Read the model definition and answer for the solid it produces. Units are mm, in the model's axes. Face numbers are marked on the shaded views. Give positions to 0.01 mm unless a question says otherwise; leave off trailing zeros. Loops run counter-clockwise (first coordinate to the right, second up) from the corner with the lowest first, then second, coordinate; pieces in that order, holes last. Notation, with made-up numbers: (14, -19.5) - (47, -19.5) arc R10 cw to (47, -4.5) - close; hole circle Ø9 at (-40, 52). An arc over 180 degrees is marked (long way). Write item = value, one per line.
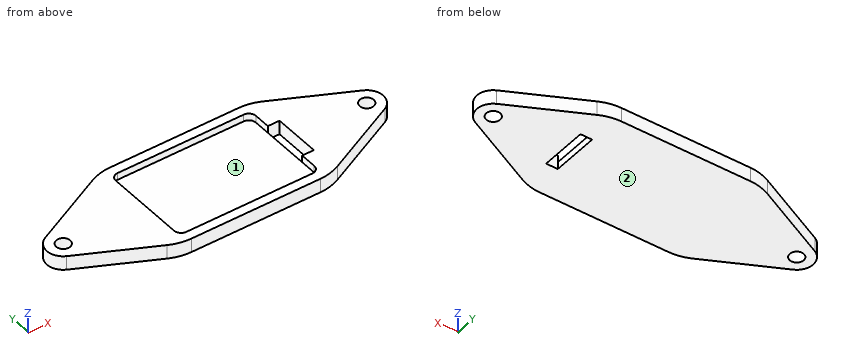
```python
from build123d import *

# Parameters (mm, degrees)
SKETCH1_R           = 1.5
BOSS_EXTRUDE1_DEPTH = 3
BOSS_EXTRUDE2_DEPTH = 1.5


with BuildPart() as part:
    # Sketch1 → Boss-Extrude1 (new body)
    with BuildSketch(Plane.XY):
        with BuildLine():
            Line((-18.151142685, 10.970518354), (-34.046738684, 3.139681424))
            ThreePointArc((-34.046738684, 3.139681424), (-35.999996343, 0.005059225), (-34.055808986, -3.135196708))
            Line((-34.055808986, -3.135196708), (-18.292240263, -10.957704881))
            ThreePointArc((-18.292240263, -10.957704881), (-16.129937386, -11.735939832), (-13.847071731, -12))
            Line((-13.847071731, -12), (13.731889302, -12))
            ThreePointArc((13.731889302, -12), (16.000679339, -11.739229526), (18.151142685, -10.970518354))
            Line((18.151142685, -10.970518354), (34.046738684, -3.139681424))
            ThreePointArc((34.046738684, -3.139681424), (35.999996343, -0.005059225), (34.055808986, 3.135196708))
            Line((34.055808986, 3.135196708), (18.292240263, 10.957704881))
            ThreePointArc((18.292240263, 10.957704881), (16.129937386, 11.735939832), (13.847071731, 12))
            Line((13.847071731, 12), (-13.731889302, 12))
            ThreePointArc((-13.731889302, 12), (-16.000679339, 11.739229526), (-18.151142685, 10.970518354))
        make_face()
        with Locations((-32.5, 0)):
            Circle(SKETCH1_R, mode=Mode.SUBTRACT)
        with BuildLine():
            Line((13.5, -10), (-13.5, -10))
            ThreePointArc((-13.5, -10), (-14.560660172, -9.560660172), (-15, -8.5))
            Line((-15, -8.5), (-15, 8.5))
            ThreePointArc((-15, 8.5), (-14.560660172, 9.560660172), (-13.5, 10))
            Line((-13.5, 10), (13.5, 10))
            ThreePointArc((13.5, 10), (14.560660172, 9.560660172), (15, 8.5))
            Line((15, 8.5), (15, 5))
            Line((15, 5), (17.5, 5))
            Line((17.5, 5), (17.5, -5))
            Line((17.5, -5), (15, -5))
            Line((15, -5), (15, -8.5))
            ThreePointArc((15, -8.5), (14.560660172, -9.560660172), (13.5, -10))
        make_face(mode=Mode.SUBTRACT)
        with Locations((32.5, 0)):
            Circle(SKETCH1_R, mode=Mode.SUBTRACT)
    extrude(amount=BOSS_EXTRUDE1_DEPTH)

    # Sketch1_3 → Boss-Extrude2 (add)
    with BuildSketch(Plane.XY):
        with BuildLine():
            Line((-13.5, 10), (13.5, 10))
            ThreePointArc((13.5, 10), (14.560660172, 9.560660172), (15, 8.5))
            Line((15, 8.5), (15, -8.5))
            ThreePointArc((15, -8.5), (14.560660172, -9.560660172), (13.5, -10))
            Line((13.5, -10), (-13.5, -10))
            ThreePointArc((-13.5, -10), (-14.560660172, -9.560660172), (-15, -8.5))
            Line((-15, -8.5), (-15, 8.5))
            ThreePointArc((-15, 8.5), (-14.560660172, 9.560660172), (-13.5, 10))
        make_face()
    extrude(amount=BOSS_EXTRUDE2_DEPTH)


solid = part.part
```
1) Each of these flat-tipped pins is pushed along its axis until it touches: P1, Ø0.8, axis at y = 1.5, z = 0.5, coming from the +X side; P2, Ø1.2, axis at y = -7.5, z = 2.5, coming from the -X side; P3, Ø3, axis at x = -1.5, y = -1.5, coming from the +Z side; P4, Ø3.5, axis at x = 32.5, y = 0, coming from the +Z side. Where does it stop, or does it pass through?
Output:
P1 = 35.82
P2 = -26.47
P3 = 1.5
P4 = 3
2) A cutting plane is placed at D-D on y = -3.75. Determine the outline of the cut face in (x, z).
Output:
outline = (-32.82, 0) - (15, 0) - (15, 1.5) - (-15, 1.5) - (-15, 3) - (-32.82, 3) - close; (17.5, 0) - (32.81, 0) - (32.81, 3) - (17.5, 3) - close
3) A cutting plane is placed at A-A on y = 0. Determine the outline of the cut face in (x, z), then the cut area to 4 significant figures.
Output:
outline = (-36, 0) - (-34, 0) - (-34, 3) - (-36, 3) - close; (-31, 0) - (15, 0) - (15, 1.5) - (-15, 1.5) - (-15, 3) - (-31, 3) - close; (17.5, 0) - (31, 0) - (31, 3) - (17.5, 3) - close; (34, 0) - (36, 0) - (36, 3) - (34, 3) - close
area = 145.5 mm²
4) Find the intervals of material crossed by probe 1 along Y at (x, z) = (-10, 2.35); probe 2 along X at (y, z) = (-0.5, 0.9); probe 3 along X at (y, z) = (-0.75, 0.45), in increasing order.
Output:
probe_1 = -12 to -10, 10 to 12
probe_2 = -35.96 to -33.91, -31.09 to 15, 17.5 to 31.09, 33.91 to 35.96
probe_3 = -35.92 to -33.8, -31.2 to 15, 17.5 to 31.2, 33.8 to 35.92
5) The mould has two halves that part along X. Classify the marked faces 1 and 2: pulls with the +X half, pulls with the -X half, needs draft (parallel to the pull), parting line crosses it, or undercut.
Output:
face_1 = undercut
face_2 = needs draft
6) A cutting plane is placed at C-C on x = -32.5. Determine the outline of the cut face in (y, z), then the cut area to 3 significant figures.
Output:
outline = (-3.91, 0) - (-1.5, 0) - (-1.5, 3) - (-3.91, 3) - close; (1.5, 0) - (3.9, 0) - (3.9, 3) - (1.5, 3) - close
area = 14.4 mm²
7) A cutting plane is placed at B-B on z = 0.65. Determine the outline of the cut face in (x, y).
Output:
outline = (-34.06, -3.14) - (-18.29, -10.96) arc R10 ccw to (-13.85, -12) - (13.73, -12) arc R10 ccw to (18.15, -10.97) - (34.05, -3.14) arc R3.5 ccw to (34.06, 3.14) - (18.29, 10.96) arc R10 ccw to (13.85, 12) - (-13.73, 12) arc R10 ccw to (-18.15, 10.97) - (-34.05, 3.14) arc R3.5 ccw to start; hole circle Ø3 at (-32.5, 0); hole (15, -5) - (17.5, -5) - (17.5, 5) - (15, 5) - close; hole circle Ø3 at (32.5, 0)
